Job drawing, mm, ordinate dimensions from the low corner. One solid piece. A direction names the side the tool comes from. Coordinates: 2 decimals unless noted, no trailing zeros. Order: outer loops, then holes, each group sorted by start corner. A loop starts at its lowest first (then second) coordinate and runs counter-clockwise, first axis right, second up. Notation, with made-up numbers: (-24, 89) - (-6, 89) arc R18 cw to (-6, 98) - close; hole circle Ø10 at (-35.5, 17). An arc over 180 degrees is marked (long way). Return JSON: item names as keys, results as strings.
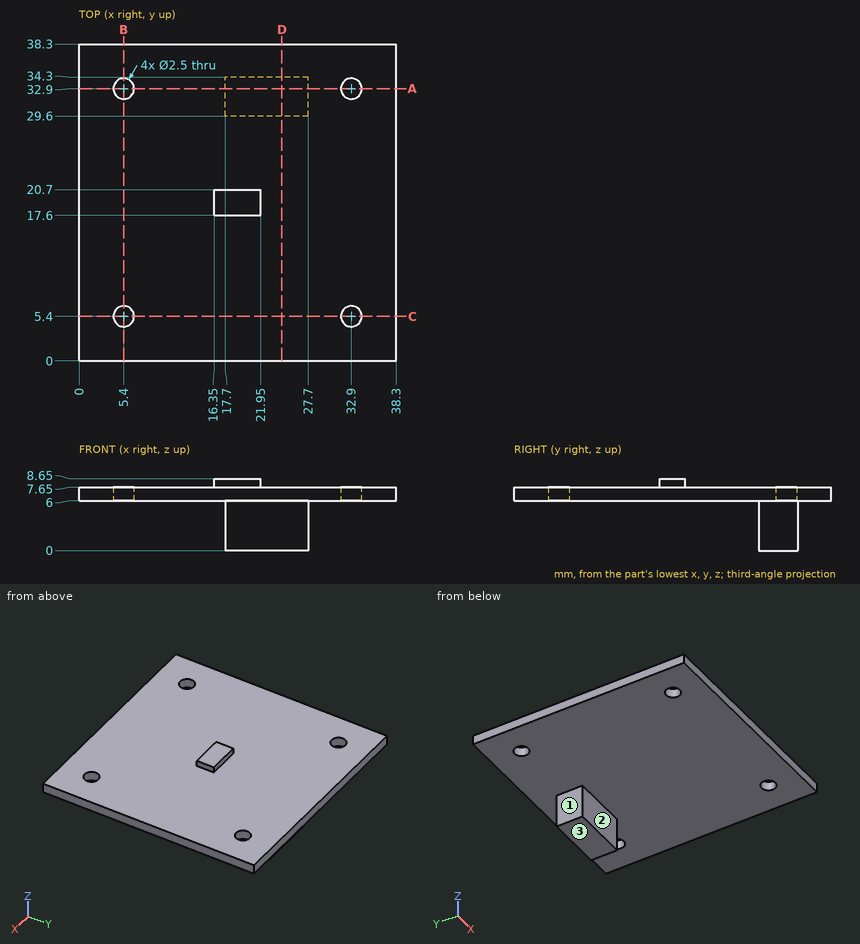
1. Cut at D-D on x = 24.5. Give the cut face in (y, z).
Check values:
{"outline": "(0, 6) - (29.6, 6) - (29.6, 0) - (34.3, 0) - (34.3, 6) - (38.3, 6) - (38.3, 7.65) - (0, 7.65) - close"}
2. Cut at B-B on x = 5.4. Give the cut face in (y, z).
Check values:
{"outline": "(0, 6) - (4.15, 6) - (4.15, 7.65) - (0, 7.65) - close; (6.65, 6) - (31.65, 6) - (31.65, 7.65) - (6.65, 7.65) - close; (34.15, 6) - (38.3, 6) - (38.3, 7.65) - (34.15, 7.65) - close"}
3. Cut at A-A on y = 32.9. Give the cut face in (x, z).
Check values:
{"outline": "(0, 6) - (4.15, 6) - (4.15, 7.65) - (0, 7.65) - close; (6.65, 6) - (17.7, 6) - (17.7, 0) - (27.7, 0) - (27.7, 6) - (31.65, 6) - (31.65, 7.65) - (6.65, 7.65) - close; (34.15, 6) - (38.3, 6) - (38.3, 7.65) - (34.15, 7.65) - close"}
4. Drop flat-ended pins along their axis: pin 1 (3 mm diameter, centred on x = 24.5, z = 3, fed in from +Y); pin 2 (0.5 mm diameter, centred on y = 19, z = 8.5, fed in from +X); pin 3 (3 mm diameter, centred on x = 5.4, y = 32.9, fed in from +Z). Give the stop position or say it passes through.
Check values:
{"pin 1": "y = 34.3", "pin 2": "x = 21.95", "pin 3": "z = 7.65"}
5. Probe L1, parallel to Y at x = 5.4, z = 7.25; L2, parallel to Z at x = 17.5, y = 13; L3, parallel to Y at x = 19.5, z = 1. List the from-to ranges inside material, lowest first.
Check values:
{"L1": "0 to 4.15, 6.65 to 31.65, 34.15 to 38.3", "L2": "6 to 7.65", "L3": "29.6 to 34.3"}
6. Tool access for the marked faces 1, 2 and 3: list every direction of +Z, -Z, +X, -X, +Y, -Y with a clear straight run to the whole face (end or side of a thin tool).
Check values:
{"face 1": "-Z, -X, +Y, -Y", "face 2": "-Z, +X, -X, -Y", "face 3": "-Z, +X, -X, +Y, -Y"}
